Check sheet for the modelled part. Datum: model origin and axes. Units: mm. A direction names the side the tool comes from. Give positions to 0.01 mm unless a question says otherwise; leave off trailing zeros. Loops run counter-clockwise (first coordinate to the right, second up) from the corner with the lowest first, then second, coordinate; pieces in that order, holes last. Notation, with made-up numbers: (82, 66.5) -> (128, 66.5) arc R8 cw to (128, 80.5) -> close; hole circle Ø4 at (41.25, -36.75). An arc over 180 degrees is marked (long way). Write each question's results on one line, items separated by ' | '. Start each with the question number.
1. Mould release check, pull along Y, two halves, no side actions. Record for faces 1 (the face through (5, 303, 25.4)), 2 (the face through (0, -9.525, 0)), 3 (the face through (9.5, 0, -3)), 4 (the face through (7.559, 132.397, 5.796)): +Y half, -Y half, draft (parallel to the pull), parting line (faces both ways), or undercut.
2. Cross-section at C-C on y = 124. Record the boundary of the cut face in (x, z) (3 decimals).
3. Cross-section at A-A on x = -6. Record the boundary of the cut face in (y, z) (3 decimals), and give its area (3 significant figures).
4. Tool access check on faces 5 (the face through (13.826, -4.696, -4.354)), 6 (the face through (-9.36, 299.49, 0.36)). Record the directions out of +Z, -Z, +X, -X, +Y, -Y that give a thin tool (end or side, any length) a straight path to the whole face; none if there is none.
5. Gauge pin test, flat ends, axial feed: pin 1 Ø12 at (x, z) = (-7.5, -8.5) entering from +Y; pin 2 Ø10 at (x, z) = (11, 17.5) entering from +Y; pin 3 Ø2 at (y, z) = (134.5, 2.5) entering from -X; pin 4 Ø1.5 at (x, y) = (-11, 192) entering from +Z (3 decimals). Record the tip position at first contact, or that the pin passes through.
6. Cross-section at B-B on z = 0. Record the boundary of the cut face in (x, y) (3 decimals), and give its area (3 significant figures).
7. Material ranges on L1, parallel to Y at x = 0, z = -15; L2, parallel to Y at x = 9.5, z = -9 (3 decimals); L3, parallel to Y at x = 0, z = -7 (3 decimals), recorded low to high. Write a range as from..to.
8. Cross-section at D-D on z = 17.5. Record the boundary of the cut face in (x, y).
Autodesk Inventor part; units mm, degrees
ref_plane "YZ Plane" through (0, 0, 0) normal (1, 0, 0) x (0, 1, 0)
ref_plane "XZ Plane" through (0, 0, 0) normal (0, 1, 0) x (-1, 0, 0)
ref_plane "XY Plane" through (0, 0, 0) normal (0, 0, 1) x (1, 0, 0)
sketch "Sketch1" plane through (0, 0, 0) normal (0, 1, 0) x (-1, 0, 0)
  circle A0 centre (0, 0) radius 9.525
  dimension "d0" = 19.05
extrude "Extrusion1" add sketch "Sketch1" along normal blind 266.7
sketch "Sketch2" plane through (0, 266.7, 0) normal (0, 1, 0) x (1, 0, 0)
  line L0 (-25.4, -25.4) -> (25.4, -25.4)
  line L1 (25.4, -25.4) -> (25.4, 25.4)
  line L2 (25.4, 25.4) -> (-25.4, 25.4)
  line L3 (-25.4, 25.4) -> (-25.4, -25.4)
  point P0 (0, 0)
extrude "Extrusion2" add sketch "Sketch2" along normal blind 50.8
sketch "Sketch3" plane through (-25.4, 266.7, 25.4) normal (0, 0, 1) x (1, 0, 0)
  circle A0 centre (25.4, 24.2057) radius 12.7
  point P0 (25.4, -266.7)
  dimension "d6" = 25.4
fillet "Fillet1" radius 25.4 4 edges at (25.4, 317.5, 0) (-25.4, 317.5, 0) (25.4, 266.7, 0) (-25.4, 266.7, 0)
extrude "Extrusion3" cut sketch "Sketch3" against normal blind 90.4875
sketch "Sketch4" plane through (0, 0, 0) normal (0, -1, 0) x (1, 0, 0)
  circle A0 centre (0, 0) radius 14.4956
extrude "Extrusion4" add sketch "Sketch4" along normal blind 9.525
properties part number "piston" material "Aluminum 6061"
Geometry says:
1) face 1: draft | face 2: -Y half | face 3: undercut | face 4: undercut
2) outline: circle Ø19.05 at (0, 0)
3) outline: (-9.525, -13.196) -> (0, -13.196) -> (0, -7.398) -> (267.419, -7.398) -> (267.419, -25.4) -> (279.712, -25.4) -> (279.712, 25.4) -> (267.419, 25.4) -> (267.419, 7.398) -> (0, 7.398) -> (0, 13.196) -> (-9.525, 13.196) -> close; (302.099, -25.4) -> (316.781, -25.4) -> (316.781, 25.4) -> (302.099, 25.4) -> close | area: 5,580 mm^2
4) face 5: -Y | face 6: +Z, -Z
5) pin 1: y = 317.46 | pin 2: y = 316.78 | pin 3: x = -9.41 | pin 4: through
6) outline: (-14.496, -9.525) -> (14.496, -9.525) -> (14.496, 0) -> (9.525, 0) -> (9.525, 268.554) arc R25.4 ccw (long way) to (-9.525, 268.554) -> (-9.525, 0) -> (-14.496, 0) -> close; hole circle Ø25.4 at (0, 290.906) | area: 6,890 mm^2
7) L1: 266.7..278.21, 303.61..317.5 | L2: -9.525..0, 268.543..282.477, 299.334..315.657 | L3: -9.525..278.206, 303.606..317.5
8) outline: circle Ø50.8 at (0, 292.1); hole circle Ø25.4 at (0, 290.91)
